```python
from build123d import *

# Parameters (mm, degrees)
F1_DEPTH = 5
F3_DEPTH = 25
F4_W     = 13.2
F4_H     = 14.5
F4_W_2   = 42
F4_H_2   = 21
F5_DEPTH = 25
F6_W     = 24
F6_H     = 21
F7_DEPTH = 5


with BuildPart() as f1:
    # F0 (on Top) → F1 (new body)
    with BuildSketch(Plane.XY):
        Polygon((44.5768064258, -65.4202470779), (44.5768064258, 49.0797529221), (-68.4231935742, 49.0797529221), (-90.9231935742, 24.5797529221), (-90.9231935742, -40.9202470779), (-68.4231935742, -65.4202470779), align=None)
    extrude(amount=F1_DEPTH)

    # F2 (on face) → F3 (join)
    with BuildSketch(Plane.XY.offset(5)):
        Polygon((-68.4231935742, -65.4202470779), (44.5768064258, -65.4202470779), (44.5768064258, 49.0797529221), (-68.4231935742, 49.0797529221), (-90.9231935742, 24.5797529221), (-90.9231935742, -40.9202470779), align=None)
        Polygon((-85.9231935742, 22.6321763094), (-66.2264395422, 44.0797529221), (39.5768064258, 44.0797529221), (39.5768064258, -60.4202470779), (-66.2264395422, -60.4202470779), (-85.9231935742, -38.9726704653), align=None, mode=Mode.SUBTRACT)
    extrude(amount=F3_DEPTH)

    # F4 (on face) → F5 (cut)
    with BuildSketch(Plane.XZ.offset(65.4202470779)):
        with Locations((-27.6231935742, 14.0335976612)):
            Rectangle(F4_W, F4_H)
        with Locations((15.9768064258, 15.5)):
            Rectangle(F4_W_2, F4_H_2)
    extrude(amount=-F5_DEPTH, mode=Mode.SUBTRACT)

    # F6 (on face) → F7 (cut, through all)
    with BuildSketch(Plane(origin=(-69.7098356481, -64.0192368197, 0), x_dir=(0.6764049996, -0.7365298884, 0), z_dir=(-0.7365298884, -0.6764049996, 0))):
        with Locations((-14.7619176963, 15.5)):
            Rectangle(F6_W, F6_H)
    extrude(amount=-F7_DEPTH, mode=Mode.SUBTRACT)


solid = f1.part
```
Source: CAD feature listing. Evaluate the final solid. Frame: model axes, mm. A direction names the side the tool comes from. Give positions to 0.01 mm unless a question says otherwise; leave off trailing zeros. Write each loop counter-clockwise with the first axis right and the second up, starting at its lowest first coordinate (ties: lowest second). Pieces come first, ordered by that corner, then holes.
1. Section query C-C (y = 16). Return the cut outline in (x, z).
2. Access query for faces 5 (the face through (-90.923, -8, 15)), 6 (the face through (-76.76, -48.95, 26.7)), 7 (the face through (-34.223, -63, 14)). Directions: +Z, -Z, +X, -X, +Y, -Y. A direction counts if a zero-diameter tool reaches every point of the face in a straight line with its end or side. Return the directions, or none.
3. First-contact query: pin 1 (5 mm diameter, centred on x = -27, y = -47, fed in from +Z); pin 2 (3 mm diameter, centred on y = 33.5, z = 20, fed in from -X); pin 3 (10 mm diameter, centred on x = -26.5, z = 15, fed in from -Y). Flat tips, straight axial feed; report the tip coordinate or a pass-through.
4. Pull-direction query (Z, two-part tool) for faces 1 (the face through (36.977, -63, 15)), 2 (the face through (-18, 47, 30)), 3 (the face through (-11, 49.08, 15)), 4 (the face through (-21.023, -63, 14)); classes: +Z half, -Z half, draft (parallel to the pull), parting line (faces both ways), or undercut.
5. Material intervals for line 1 along Y through (x, z) = (-46, 11.5); line 2 along Z through (x, y) = (-83.5, -45.5); line 3 along X through (y, z) = (-15.5, 9), sorted ascending.
6. Section query B-B (z = 11.5). Return the cut outline in (x, y) (3 decimals), then the cut area to 3 significant figures.
7. Section query A-A (x = 2). Return the cut outline in (y, z).
8. Section query D-D (x = -14). Return the cut outline in (y, z), then the cut area to 4 significant figures.
Output values:
1. outline: (-90.92, 0) - (44.58, 0) - (44.58, 30) - (39.58, 30) - (39.58, 5) - (-85.92, 5) - (-85.92, 30) - (-90.92, 30) - close
2. face 5: +Z, -Z, -X, +Y, -Y
2. face 6: +Z
2. face 7: -Y
3. pin 1: stops at z = 5
3. pin 2: stops at x = -84.11
3. pin 3: stops at y = 44.08
4. face 1: undercut
4. face 2: +Z half
4. face 3: draft
4. face 4: undercut
5. line 1: y = -65.42 to -60.42, 44.08 to 49.08
5. line 2: z = 0 to 5, 26 to 30
5. line 3: x = -90.92 to -85.92, 39.58 to 44.58
6. outline: (-90.923, -40.92) - (-87.812, -44.308) - (-84.129, -40.926) - (-85.923, -38.973) - (-85.923, 22.632) - (-66.226, 44.08) - (39.577, 44.08) - (39.577, -60.42) - (36.977, -60.42) - (36.977, -65.42) - (44.577, -65.42) - (44.577, 49.08) - (-68.423, 49.08) - (-90.923, 24.58) - close; (-71.578, -61.985) - (-68.423, -65.42) - (-34.223, -65.42) - (-34.223, -60.42) - (-66.226, -60.42) - (-67.895, -58.603) - close; (-21.023, -65.42) - (-5.023, -65.42) - (-5.023, -60.42) - (-21.023, -60.42) - close
6. area: 1,880 mm2
7. outline: (-65.42, 0) - (49.08, 0) - (49.08, 30) - (44.08, 30) - (44.08, 5) - (-65.42, 5) - close; (-65.42, 26) - (-60.42, 26) - (-60.42, 30) - (-65.42, 30) - close
8. outline: (-65.42, 0) - (49.08, 0) - (49.08, 30) - (44.08, 30) - (44.08, 5) - (-60.42, 5) - (-60.42, 30) - (-65.42, 30) - close
8. area: 822.5 mm2
